```python
from build123d import *

# Parameters (mm, degrees)
SKETCH1_W           = 160
SKETCH1_H           = 160
BOSS_EXTRUDE1_DEPTH = 75
SKETCH2_W           = 150
SKETCH2_H           = 150
CUT_EXTRUDE1_DEPTH  = 65
SKETCH3_W           = 15
SKETCH3_H           = 65
BOSS_EXTRUDE2_DEPTH = 15
SKETCH4_W           = 10
SKETCH4_H           = 65
BOSS_EXTRUDE3_DEPTH = 10
FILLET1_R           = 10
SKETCH11_W          = 25
SKETCH11_H          = 65
BOSS_EXTRUDE4_DEPTH = 5
FILLET2_R           = 30
SKETCH15_R          = 1.5
CUT_EXTRUDE2_DEPTH  = 10
SKETCH17_R          = 3
CUT_EXTRUDE3_DEPTH  = 1.5
SKETCH18_W          = 10
SKETCH18_H          = 145
CUT_EXTRUDE6_DEPTH  = 5


with BuildPart() as part:
    # Sketch1 → Boss-Extrude1 (new body)
    with BuildSketch(Plane(origin=(0, 0, 0), x_dir=(1, 0, 0), z_dir=(0, 1, 0))):
        Rectangle(SKETCH1_W, SKETCH1_H)
    extrude(amount=BOSS_EXTRUDE1_DEPTH)

    # Sketch2 → Cut-Extrude1 (cut)
    with BuildSketch(Plane(origin=(0, 75, 0), x_dir=(1, 0, 0), z_dir=(0, 1, 0))):
        with Locations((0, 5)):
            Rectangle(SKETCH2_W, SKETCH2_H)
    extrude(amount=-CUT_EXTRUDE1_DEPTH, mode=Mode.SUBTRACT)

    # Sketch3 → Boss-Extrude2 (add)
    with BuildSketch(Plane(origin=(0, 0, 70), x_dir=(-1, 0, 0), z_dir=(0, 0, -1))):
        with Locations((-67.5, 42.5)):
            Rectangle(SKETCH3_W, SKETCH3_H)
        with Locations((67.5, 42.5)):
            Rectangle(SKETCH3_W, SKETCH3_H)
    extrude(amount=BOSS_EXTRUDE2_DEPTH)

    # Sketch4 → Boss-Extrude3 (add)
    with BuildSketch(Plane(origin=(0, 0, 70), x_dir=(-1, 0, 0), z_dir=(0, 0, -1))):
        with Locations((-55, 42.5)):
            Rectangle(SKETCH4_W, SKETCH4_H)
        with Locations((55, 42.5)):
            Rectangle(SKETCH4_W, SKETCH4_H)
    extrude(amount=BOSS_EXTRUDE3_DEPTH)

    # Fillet1
    fillet1_edges = [part.edges().sort_by_distance(p)[0] for p in [
        (80, 37.5, 80),
        (-80, 37.5, 80),
    ]]
    fillet(fillet1_edges, radius=FILLET1_R)

    # Sketch11 → Boss-Extrude4 (add)
    with BuildSketch(Plane(origin=(0, 0, 70), x_dir=(-1, 0, 0), z_dir=(0, 0, -1))):
        with Locations((-37.5, 42.5)):
            Rectangle(SKETCH11_W, SKETCH11_H)
        with Locations((37.5, 42.5)):
            Rectangle(SKETCH11_W, SKETCH11_H)
    extrude(amount=BOSS_EXTRUDE4_DEPTH)

    # Fillet2
    fillet2_edges = [part.edges().sort_by_distance(p)[0] for p in [
        (-77.5, 75, -80),
        (77.5, 75, -80),
    ]]
    fillet(fillet2_edges, radius=FILLET2_R)

    # Sketch15 → Cut-Extrude2 (cut)
    with BuildSketch(Plane.XZ):
        with Locations((-60, 10)):
            Circle(SKETCH15_R)
        with Locations((-40, 10)):
            Circle(SKETCH15_R)
        with Locations((40, 10)):
            Circle(SKETCH15_R)
        with Locations((60, 10)):
            Circle(SKETCH15_R)
        with Locations((60, -10)):
            Circle(SKETCH15_R)
        with Locations((40, -10)):
            Circle(SKETCH15_R)
        with Locations((-40, -10)):
            Circle(SKETCH15_R)
        with Locations((-60, -10)):
            Circle(SKETCH15_R)
    extrude(amount=-CUT_EXTRUDE2_DEPTH, mode=Mode.SUBTRACT)

    # Sketch17 → Cut-Extrude3 (cut)
    with BuildSketch(Plane(origin=(0, 10, 0), x_dir=(1, 0, 0), z_dir=(0, 1, 0))):
        with Locations((-60, 10)):
            Circle(SKETCH17_R)
        with Locations((-40, 10)):
            Circle(SKETCH17_R)
        with Locations((-40, -10)):
            Circle(SKETCH17_R)
        with Locations((-60, -10)):
            Circle(SKETCH17_R)
        with Locations((40, -10)):
            Circle(SKETCH17_R)
        with Locations((60, -10)):
            Circle(SKETCH17_R)
        with Locations((40, 10)):
            Circle(SKETCH17_R)
        with Locations((60, 10)):
            Circle(SKETCH17_R)
    extrude(amount=-CUT_EXTRUDE3_DEPTH, mode=Mode.SUBTRACT)

    # Sketch18 → Cut-Extrude6 (cut)
    with BuildSketch(Plane(origin=(0, 10, 0), x_dir=(1, 0, 0), z_dir=(0, 1, 0))):
        with Locations((10, 7.5)):
            Rectangle(SKETCH18_W, SKETCH18_H)
        with Locations((-10, 7.5)):
            Rectangle(SKETCH18_W, SKETCH18_H)
    extrude(amount=-CUT_EXTRUDE6_DEPTH, mode=Mode.SUBTRACT)


solid = part.part
```
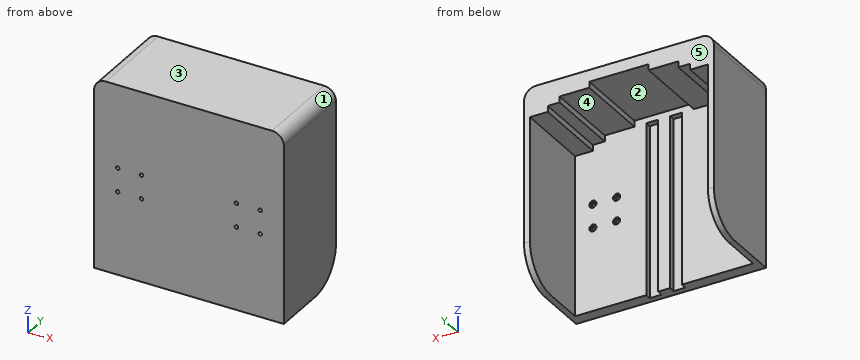
Geometry: final body of the model. Coordinates: model frame, mm. Face numbers are marked on the shaded views. A direction names the side the tool comes from. Coordinates: 2 decimals unless noted, no trailing zeros. Order: outer loops, then holes, each group sorted by start corner. A loop starts at its lowest first (then second) coordinate and runs counter-clockwise, first axis right, second up. Notation, with made-up numbers: (-2.75, -40) - (13.25, -40) arc R4 cw to (13.25, -33) - close; hole circle Ø1 at (22, 44.5). An arc over 180 degrees is marked (long way). Return JSON: item names as keys, results as strings. Group by question number.
1. Cut plane C-C (x = 3). Output: boundary loops of the cut face in (y, z).
2. Cut plane B-B (y = 13). Output: boundary loops of the cut face in (x, z).
3. Pull-direction query (X, two-part tool) for the marked faces 1, 2 and 3; classes: pulls with the +X half, pulls with the -X half, needs draft (parallel to the pull), parting line crosses it, or undercut.
4. Material intervals for line 1 along Z through (x, y) = (-40, 9.4); line 2 along Z through (x, y) = (-60, 4); line 3 along X through (y, z) = (9, -38), sorted ascending. Write a range as [from, to].
5. Cut plane D-D (z = 58). Output: boundary loops of the cut face in (x, y), plus the area to 3 significant figures.
6. Pin query (flat end, axial travel): pin 1 (3 mm diameter, centred on x = 55, z = -49, fed in from +Y); pin 2 (4 mm diameter, centred on x = -5, y = 36, fed in from -Z); pin 3 (2.5 mm diameter, centred on x = 60, z = 10, fed in from -Y); pin 4 (2 mm diameter, centred on x = -41.5, z = -61, fed in from -Y). Return the tip coordinate at first contact, or that it passes through.
7. Set-up query: the marked faces 4 and 5. Return all of +Z, -Z, +X, -X, +Y, -Y with unobstructed straight access to the full face (end or side cutting, diameter ignored); none if empty.
8. Cut plane A-A (z = -25). Output: boundary loops of the cut face in (x, y), plus the area to 3 significant figures.
Resolved:
{
 "1": {"outline": "(0, -80) - (10, -80) - (10, 70) - (75, 70) - (75, 80) - (0, 80) - close"},
 "2": {"outline": "(-80, -80) - (-75, -80) - (-75, 55) - (-60, 55) - (-60, 60) - (-50, 60) - (-50, 65) - (-25, 65) - (-25, 70) - (25, 70) - (25, 65) - (50, 65) - (50, 60) - (60, 60) - (60, 55) - (75, 55) - (75, -80) - (80, -80) - (80, 70) arc R10 ccw to (70, 80) - (-70, 80) arc R10 ccw to (-80, 70) - close"},
 "3": {"face 1": "pulls with the +X half", "face 2": "undercut", "face 3": "needs draft"},
 "4": {"line 1": "z = [-80, -13], [-7, 7], [13, 80]", "line 2": "z = [-80, -11.5], [-8.5, 8.5], [11.5, 80]", "line 3": "x = [-80, -15], [-5, 5], [15, 80]"},
 "5": {"outline": "(-80, 0) - (80, 0) - (80, 75) - (60, 75) - (60, 10) - (15, 10) - (15, 5) - (5, 5) - (5, 10) - (-5, 10) - (-5, 5) - (-15, 5) - (-15, 10) - (-60, 10) - (-60, 75) - (-80, 75) - close", "area": "4,100 mm²"},
 "6": {"pin 1": "stops at y = 10", "pin 2": "stops at z = 70", "pin 3": "passes through", "pin 4": "stops at y = 0"},
 "7": {"face 4": "-Z, +Y", "face 5": "+Z, -Z, +X, -X, +Y"},
 "8": {"outline": "(-80, 0) - (80, 0) - (80, 75) - (75, 75) - (75, 10) - (15, 10) - (15, 5) - (5, 5) - (5, 10) - (-5, 10) - (-5, 5) - (-15, 5) - (-15, 10) - (-75, 10) - (-75, 75) - (-80, 75) - close", "area": "2,150 mm²"}
}
